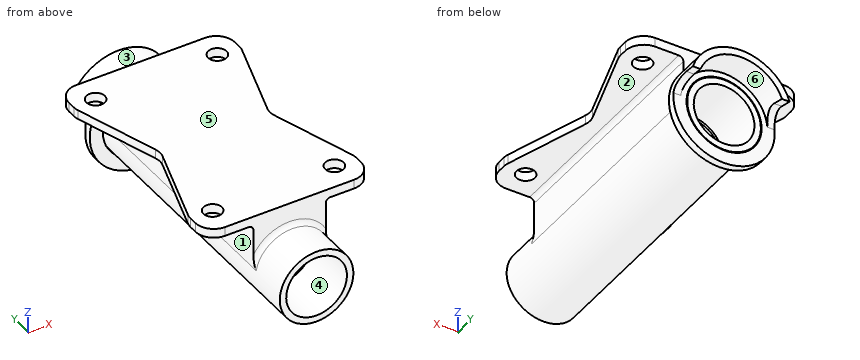
from build123d import *
from build123d.topology import SkipClean

# Parameters (mm, degrees)
BOSS_EXTRUDE1_DEPTH      = 3.175
BOSS_EXTRUDE4_START      = 150.025
BOSS_EXTRUDE4_DEPTH      = 150.025
BOSS_EXTRUDE5_START      = 3.175
BOSS_EXTRUDE5_DEPTH      = 3.175
SKETCH18_W               = 114.3
SKETCH18_H               = 173.2
BOSS_EXTRUDE6_DEPTH      = 6.35
BOSS_EXTRUDE9_DEPTH      = 1.5875
BOSS_EXTRUDE9_DEPTH_BACK = 1.5875
SKETCH26_R               = 35
SKETCH26_R_2             = 25.899999994
BOSS_EXTRUDE7_DEPTH      = 5
BOSS_EXTRUDE8_DEPTH      = 19.05
CUT_EXTRUDE3_DEPTH       = 231.866297886
CUT_EXTRUDE3_DEPTH_BACK  = 231.866297886
BOSS_EXTRUDE10_START     = 150.025
BOSS_EXTRUDE10_DEPTH     = 150.025
BOSS_EXTRUDE11_START     = 9.325
BOSS_EXTRUDE11_DEPTH     = 9.325
SKETCH36_W               = 6.35
SKETCH36_H               = 7.5
CUT_EXTRUDE4_DEPTH       = 252.192386516
FILLET1_R                = 3.175
CUT_EXTRUDE5_DEPTH       = 238.723253055
FILLET2_R                = 12.7
SKETCH38_R               = 6.35
CUT_EXTRUDE6_DEPTH       = 238.723253055
SKETCH41_R               = 25.399999994
CUT_EXTRUDE8_DEPTH       = 213.813709708


with BuildPart() as part:
    # Sketch12 → Revolve1 (revolve)
    with BuildSketch(Plane.XY, mode=Mode.PRIVATE) as revolve1_sk:
        Polygon((-25.399999994, 0), (-25.399999994, 203.2), (-20.955, 203.2), (-20.955, 165.1), (-19.177, 165.1), (-19.177, 38.1), (-20.955, 38.1), (-20.955, 0), align=None)
    revolve(revolve1_sk.sketch.rotate(Axis((0, 0, 0), (0, 1, 0)), 270), axis=Axis((0, 0, 0), (0, 1, 0)))



with BuildPart() as body_2:
    # Sketch14 → Boss-Extrude1 (new body)
    with BuildSketch(Plane(origin=(0, 30, 0), x_dir=(-1, 0, 0), z_dir=(0, -1, 0))):
        with BuildLine():
            Line((-25, -4.489988829), (-25, -35.399999994))
            Line((-25, -35.399999994), (25, -35.399999994))
            Line((25, -35.399999994), (25, -4.489988829))
            ThreePointArc((25, -4.489988829), (0, -25.399999994), (-25, -4.489988829))
        make_face()
    extrude(amount=-BOSS_EXTRUDE1_DEPTH)

    # Sketch15 → Boss-Extrude4 (add)
    with BuildSketch(Plane(origin=(0, 33.175, 0), x_dir=(1, 0, 0), z_dir=(0, 1, 0)).offset(BOSS_EXTRUDE4_START)):
        with BuildLine():
            Line((-1.5875, -25.350342077), (-1.5875, -35.399999994))
            Line((-1.5875, -35.399999994), (1.5875, -35.399999994))
            Line((1.5875, -35.399999994), (1.5875, -25.350342077))
            ThreePointArc((1.5875, -25.350342077), (0, -25.399999994), (-1.5875, -25.350342077))
        make_face()
    extrude(amount=-BOSS_EXTRUDE4_DEPTH)

    # Sketch17 → Boss-Extrude5 (add)
    with BuildSketch(Plane(origin=(0, 183.2, 0), x_dir=(1, 0, 0), z_dir=(0, 1, 0)).offset(BOSS_EXTRUDE5_START)):
        with BuildLine():
            Line((25, -35.399999994), (25, -4.489988829))
            ThreePointArc((25, -4.489988829), (0, -25.399999994), (-25, -4.489988829))
            Line((-25, -4.489988829), (-25, -35.399999994))
            Line((-25, -35.399999994), (25, -35.399999994))
        make_face()
    extrude(amount=-BOSS_EXTRUDE5_DEPTH)

    # Sketch18 → Boss-Extrude6 (add)
    with BuildSketch(Plane.XY.offset(35.399999994)):
        with Locations((0, 116.6)):
            Rectangle(SKETCH18_W, SKETCH18_H)
    extrude(amount=BOSS_EXTRUDE6_DEPTH)


with BuildPart() as part_1:
    add(part.part)

    add(body_2.part)  # Boss-Extrude9 merges body 2
    # Sketch30 → Boss-Extrude9 (add, two sides: drawn at the far end of the back side and taken through both)
    with BuildSketch(Plane(origin=(0, 106.6, 0), x_dir=(-1, 0, 0), z_dir=(0, -1, 0)).offset(-BOSS_EXTRUDE9_DEPTH_BACK)):
        with BuildLine():
            Line((25, -35.399999994), (25, -4.489988829))
            ThreePointArc((25, -4.489988829), (0, -25.399999994), (-25, -4.489988829))
            Line((-25, -4.489988829), (-25, -35.399999994))
            Line((-25, -35.399999994), (25, -35.399999994))
        make_face()
    extrude(amount=BOSS_EXTRUDE9_DEPTH + BOSS_EXTRUDE9_DEPTH_BACK)


with BuildPart() as body_2_2:
    # Sketch26 → Boss-Extrude7 (new body)
    with BuildSketch(Plane(origin=(0, 200.7, 0), x_dir=(1, 0, 0), z_dir=(0, 1, 0))):
        with Locations(Location((0, 0, 0), (0, 0, 270))):
            Circle(SKETCH26_R)
        with Locations(Location((0, 0, 0), (0, 0, 270))):
            Circle(SKETCH26_R_2, mode=Mode.SUBTRACT)
    extrude(amount=-BOSS_EXTRUDE7_DEPTH)

    # Sketch26<3> → Boss-Extrude8 (add)
    with SkipClean():  # the faces are left unmerged after this step: merging them gives an invalid solid
        with BuildSketch(Plane(origin=(0, 200.7, 0), x_dir=(1, 0, 0), z_dir=(0, 1, 0))):
            with BuildLine():
                ThreePointArc((-34.910600109, -2.5), (0, -35), (34.910600109, -2.5))
                Line((34.910600109, -2.5), (29.895651858, -2.5))
                ThreePointArc((29.895651858, -2.5), (0, -30), (-29.895651858, -2.5))
                Line((-29.895651858, -2.5), (-34.910600109, -2.5))
            make_face()
        extrude(amount=BOSS_EXTRUDE8_DEPTH)


with BuildPart() as cut_extrude3_tool:
    # Sketch33 → Cut-Extrude3 (new, two sides: drawn at the far end of the back side and taken through both)
    with SkipClean():  # the faces are left unmerged after this step: merging them gives an invalid solid
        with BuildSketch(Plane(origin=(0, 0, 0), x_dir=(0, 0, -1), z_dir=(1, 0, 0)).offset(-CUT_EXTRUDE3_DEPTH_BACK)):
            with BuildLine():
                Line((-2.5, 219.75), (-2.99214107, 219.75))
                Line((-2.99214107, 219.75), (-10.5, 219.75))
                Line((-10.5, 219.75), (-11.8865543, 211.886459809))
                ThreePointArc((-11.8865543, 211.886459809), (-9.801443088, 204.104718827), (-2.5, 200.7))
                Line((-2.5, 200.7), (-2.5, 219.75))
            make_face()
        extrude(amount=CUT_EXTRUDE3_DEPTH + CUT_EXTRUDE3_DEPTH_BACK)


with BuildPart() as part_2:
    with SkipClean():  # the faces are left unmerged after this step: merging them gives an invalid solid
        add(part_1.part)

        # Cut-Extrude3: cut by cut_extrude3_tool
        add(cut_extrude3_tool.part, mode=Mode.SUBTRACT)

    # Sketch34 → Boss-Extrude10 (add)
    with BuildSketch(Plane(origin=(0, 33.175, 0), x_dir=(1, 0, 0), z_dir=(0, 1, 0)).offset(BOSS_EXTRUDE10_START)):
        with BuildLine():
            Line((-25, -35.399999994), (-1.5875, -35.399999994))
            Line((-1.5875, -35.399999994), (-1.5875, -25.350342077))
            ThreePointArc((-1.5875, -25.350342077), (-16.897111394, -18.964377823), (-25, -4.489988829))
            Line((-25, -4.489988829), (-25, -35.399999994))
        make_face()
        with BuildLine():
            Line((1.5875, -25.350342077), (1.5875, -35.399999994))
            Line((1.5875, -35.399999994), (25, -35.399999994))
            Line((25, -35.399999994), (25, -4.489988829))
            ThreePointArc((25, -4.489988829), (16.897111394, -18.964377823), (1.5875, -25.350342077))
        make_face()
    extrude(amount=-BOSS_EXTRUDE10_DEPTH)



with BuildPart() as body_2_2_1:
    with SkipClean():  # the faces are left unmerged after this step: merging them gives an invalid solid
        add(body_2_2.part)

        # Cut-Extrude3: cut by cut_extrude3_tool
        add(cut_extrude3_tool.part, mode=Mode.SUBTRACT)


with BuildPart() as part_3:
    with SkipClean():  # the faces are left unmerged after this step: merging them gives an invalid solid
        add(part_2.part)

        add(body_2_2_1.part)  # Boss-Extrude11 merges body 2 2
        # Sketch35 → Boss-Extrude11 (add)
        with BuildSketch(Plane(origin=(0, 186.375, 0), x_dir=(1, 0, 0), z_dir=(0, 1, 0)).offset(BOSS_EXTRUDE11_START)):
            with BuildLine():
                Line((-25, -35.399999994), (25, -35.399999994))
                Line((25, -35.399999994), (25, -4.489988829))
                ThreePointArc((25, -4.489988829), (0, -25.399999994), (-25, -4.489988829))
                Line((-25, -4.489988829), (-25, -35.399999994))
            make_face()
        extrude(amount=-BOSS_EXTRUDE11_DEPTH)

    # Sketch36 → Cut-Extrude4 (cut, through all)
    with SkipClean():  # the faces are left unmerged after this step: merging them gives an invalid solid
        with BuildSketch(Plane(origin=(57.15, 0, 0), x_dir=(0, 0, -1), z_dir=(1, 0, 0))):
            with Locations((-38.574999994, 199.45)):
                Rectangle(SKETCH36_W, SKETCH36_H)
        extrude(amount=-CUT_EXTRUDE4_DEPTH, mode=Mode.SUBTRACT)

    # Fillet1
    fillet1_edges = [part_3.edges().sort_by_distance(p)[0] for p in [
        (-25, 112.85, 35.399999994),
        (25, 112.85, 35.399999994),
        (0, 30, 25.399999994),
    ]]
    fillet(fillet1_edges, radius=FILLET1_R)

    # Sketch37 → Cut-Extrude5 (cut, through all)
    with SkipClean():  # the faces are left unmerged after this step: merging them gives an invalid solid
        with BuildSketch(Plane(origin=(0, 0, 35.399999994), x_dir=(-1, 0, 0), z_dir=(0, 0, -1))):
            Polygon((-57.15, 175.7), (-37.333471119, 112.85), (-57.15, 50), align=None)
            Polygon((57.15, 50), (37.333471119, 112.85), (57.15, 175.7), align=None)
        extrude(amount=-CUT_EXTRUDE5_DEPTH, mode=Mode.SUBTRACT)

    # Fillet2
    fillet2_edges = [part_3.edges().sort_by_distance(p)[0] for p in [
        (-57.15, 195.7, 38.574999994),
        (57.15, 195.7, 38.574999994),
        (-57.15, 50, 38.574999994),
        (-37.333471119, 112.85, 38.574999994),
        (-57.15, 175.7, 38.574999994),
        (37.333471119, 112.85, 38.574999994),
        (57.15, 50, 38.574999994),
        (57.15, 175.7, 38.574999994),
        (-57.15, 30, 38.574999994),
        (57.15, 30, 38.574999994),
    ]]
    fillet(fillet2_edges, radius=FILLET2_R)

    # Sketch38 → Cut-Extrude6 (cut, through all)
    with SkipClean():  # the faces are left unmerged after this step: merging them gives an invalid solid
        with BuildSketch(Plane(origin=(0, 0, 35.399999994), x_dir=(-1, 0, 0), z_dir=(0, 0, -1))):
            with Locations((-42, 177.85)):
                Circle(SKETCH38_R)
            with Locations(Location((42, 177.85, 0), (0, 0, 180))):
                Circle(SKETCH38_R)
            with Locations((42, 47.85)):
                Circle(SKETCH38_R)
            with Locations(Location((-42, 47.85, 0), (0, 0, 180))):
                Circle(SKETCH38_R)
        extrude(amount=-CUT_EXTRUDE6_DEPTH, mode=Mode.SUBTRACT)

    # Sketch41 → Cut-Extrude8 (cut, through all)
    with SkipClean():  # the faces are left unmerged after this step: merging them gives an invalid solid
        with BuildSketch(Plane(origin=(0, 200.7, 0), x_dir=(1, 0, 0), z_dir=(0, 1, 0))):
            with Locations(Location((0, 0, 0), (0, 0, 90))):
                Circle(SKETCH41_R)
        extrude(amount=CUT_EXTRUDE8_DEPTH, mode=Mode.SUBTRACT)


solid = part_3.part
Geometry check sheet. Reference: the model listing, model coordinates, mm. Face numbers are marked on the shaded views. A direction names the side the tool comes from. Give positions to 0.01 mm unless a question says otherwise; leave off trailing zeros. Order: outer loops, then holes, each group sorted by start corner. A loop starts at its lowest first (then second) coordinate and runs counter-clockwise, first axis right, second up. Notation, with made-up numbers: (-26, 85.5) - (28, 85.5) arc R19 ccw to (28, 91.5) - close; hole circle Ø11 at (3, 56.5). An arc over 180 degrees is marked (long way). Use one line per item in the form item = value.
1) Sectioned sample at A-A (z = 0). Record the boundary of the cut face in (x, y) (3 decimals), and give its area (3 significant figures).
Working result:
outline = (-35, 195.7) - (-25.9, 195.7) - (-25.9, 200.7) - (-35, 200.7) - close; (-25.4, 0) - (-20.955, 0) - (-20.955, 38.1) - (-19.177, 38.1) - (-19.177, 165.1) - (-20.955, 165.1) - (-20.955, 200.7) - (-25.4, 200.7) - close; (19.177, 38.1) - (20.955, 38.1) - (20.955, 0) - (25.4, 0) - (25.4, 200.7) - (20.955, 200.7) - (20.955, 165.1) - (19.177, 165.1) - close; (25.9, 195.7) - (35, 195.7) - (35, 200.7) - (25.9, 200.7) - close
area = 2,330 mm^2
2) Access from +Z, -Z, +X, -X, +Y, -Y to the whole of each face (thin tool, end or side, straight path). Record for the marked faces 1, 2 and 3.
Working result:
face_1 = -X, -Y
face_2 = -Z, +X, +Y, -Y
face_3 = +Y
3) Sectioned sample at C-C (z = 37.5). Record the boundary of the cut face in (x, y), and give its area (3 significant figures).
Working result:
outline = (-57.15, 42.7) arc R12.7 ccw to (-44.45, 30) - (44.45, 30) arc R12.7 ccw to (57.15, 42.7) - (57.15, 48.05) arc R12.7 ccw to (56.56, 51.86) - (38.54, 109.03) arc R12.7 cw to (38.54, 116.67) - (56.56, 173.84) arc R12.7 ccw to (57.15, 177.65) - (57.15, 183) arc R12.7 ccw to (44.45, 195.7) - (-44.45, 195.7) arc R12.7 ccw to (-57.15, 183) - (-57.15, 177.65) arc R12.7 ccw to (-56.56, 173.84) - (-38.54, 116.67) arc R12.7 cw to (-38.54, 109.03) - (-56.56, 51.86) arc R12.7 ccw to (-57.15, 48.05) - close; hole circle Ø12.7 at (-42, 47.85); hole circle Ø12.7 at (-42, 177.85); hole circle Ø12.7 at (42, 47.85); hole circle Ø12.7 at (42, 177.85)
area = 15,800 mm^2
4) Depth check by flat-ended pin: pin 1 Ø12 at (x, y) = (32, 80) entering from -Z; pin 2 Ø12.5 at (x, z) = (9.5, 3.5) entering from +Y; pin 3 Ø10 at (y, z) = (65.5, -2.5) entering from +X; pin 4 Ø14 at (y, z) = (122, 13.5) entering from +X. Enter the tip coordinate at first touch or a pass-through.
Working result:
pin_1 = 34.54
pin_2 = through
pin_3 = 25.4
pin_4 = 25
5) Draft check along Z on the marked faces 4, 5 and 6. Enter one of: released by +Z, released by -Z, zero draft, split by the parting line, or undercut.
Working result:
face_4 = undercut
face_5 = released by +Z
face_6 = released by -Z
6) Material ranges on probe 1 along X at (y, z) = (9, 0) (3 decimals); probe 2 along X at (y, z) = (198, 0) (3 decimals); probe 3 along X at (y, z) = (196.5, -16), recorded low to high. Write a range as from..to.
Working result:
probe_1 = -25.4..-20.955, 20.955..25.4
probe_2 = -35..-25.9, -25.4..-20.955, 20.955..25.4, 25.9..35
probe_3 = -31.13..-20.37, -19.73..-13.53, 13.53..19.73, 20.37..31.13
7) Sectioned sample at D-D (y = 143). Record the boundary of the cut face in (x, z) (3 decimals).
Working result:
outline = (-46.84, 35.4) - (-28.175, 35.4) arc R3.175 cw to (-25, 32.225) - (-25, 4.49) arc R25.4 ccw (long way) to (25, 4.49) - (25, 32.225) arc R3.175 cw to (28.175, 35.4) - (46.84, 35.4) - (46.84, 41.75) - (-46.84, 41.75) - close; hole circle Ø38.354 at (0, 0)
8) Sectioned sample at B-B (x = 0). Count the separate pieces of the cut face and the enclosed holes in it, and give its area (3 significant figures).
Working result:
separate_pieces = 3
enclosed_holes = 0
area = 5,130 mm^2
